```python
from build123d import *

# Parameters (mm, degrees)
BOX_W             = 5
BOX_H             = 6
BOX_DEPTH         = 8
CYLINDER001_R     = 1.675
CYLINDER001_DEPTH = 8


with BuildPart() as d:
    # Box → Box (new body)
    with BuildSketch(Plane(origin=(1, -3, 15), x_dir=(1, 0, 0), z_dir=(0, 0, 1))):
        with Locations((2.5, 3)):
            Rectangle(BOX_W, BOX_H)
    extrude(amount=BOX_DEPTH)


with BuildPart() as eje_d:
    # Cylinder001 → Cylinder001 (new body)
    with BuildSketch(Plane.XY.offset(15)):
        Circle(CYLINDER001_R)
    extrude(amount=CYLINDER001_DEPTH)

    # Cut: cut D
    add(d.part, mode=Mode.SUBTRACT)


with BuildPart() as eje_d_1:
    # Cut placement: moved
    add(eje_d.part.moved(Location((0, 0, -12))))


with BuildPart() as cut001:
    # Sketch → Revolution (revolve)
    with BuildSketch(Plane.XZ):
        Polygon((9.5, 11), (0, 11), (0, 0), (9.5, 0), (9.5, 0.5), (10, 0.5), (10, 10.5), (9.5, 10.5), align=None)
    revolve(axis=Axis((0, 0, 0), (0, 0, 1)))

    # Cut001: cut EJE + D
    add(eje_d_1.part, mode=Mode.SUBTRACT)


solid = cut001.part
```
Check sheet for the modelled part. Datum: model origin and axes. Units: mm. A direction names the side the tool comes from. Give positions to 0.01 mm unless a question says otherwise; leave off trailing zeros. Order: outer loops, then holes, each group sorted by start corner. A loop starts at its lowest first (then second) coordinate and runs counter-clockwise, first axis right, second up. Notation, with made-up numbers: (66.5, -5) -> (79.5, -5) arc R25 ccw to (79.5, 23) -> close; hole circle Ø5 at (-34, 1.5). An arc over 180 degrees is marked (long way). Return JSON: item names as keys, results as strings.
1. Set-up check for faces 5 (the flat face through (0, 0, 3)), 6 (the cylindrical face through (4.38, -8.43, 0.25)), 7 (the cylindrical face through (-2.17, -9.76, 5.57)): record each of +Z, -Z, +X, -X, +Y, -Y from which the full face is reachable in a straight line by a thin tool's end or side.
From the geometry:
{"face 5": "+Z", "face 6": "-Z", "face 7": "+Z, -Z"}
2. Mould release check, pull along Y, two halves, no side actions. Record for faces 1 (the flat face through (1, 0, 7)), 2 (the cylindrical face through (-1.674, 0.052, 6.944)), 3 (the flat face through (0, 0, 0)), 4 (the cylindrical face through (4.38, -8.43, 10.75)): +Y half, -Y half, draft (parallel to the pull), parting line (faces both ways), or undercut.
From the geometry:
{"face 1": "undercut", "face 2": "undercut", "face 3": "draft", "face 4": "parting line"}
3. Material ranges on probe 1 along Y at (x, z) = (0, 8) (3 decimals); probe 2 along X at (y, z) = (-2.25, 4); probe 3 along Y at (x, z) = (3, 3.5), recorded low to high. Write a range as [from, to].
From the geometry:
{"probe 1": "[-10, -1.675], [1.675, 10]", "probe 2": "[-9.74, 9.74]", "probe 3": "[-9.54, 9.54]"}
4. Cross-section at C-C, the plane z = 8.25. Record the cut outline in (x, y) (3 decimals).
From the geometry:
{"outline": "circle Ø20 at (0, 0); hole (1, -1.344) -> (1, 1.344) arc R1.675 ccw (long way) to start"}
5. Go/stop test with flat-tipped pins: P1, Ø5, axis at y = -3.5, z = 6.5, coming from the -X side; P2, Ø5, axis at x = 3, z = 3.5, coming from the -Y side; P3, Ø1, axis at x = -3.5, z = 2.5, coming from the +Y side. Record where each tip stops, or that it passes through.
From the geometry:
{"P1": "x = -9.95", "P2": "y = -9.99", "P3": "y = 9.54"}
6. Cross-section at D-D, the plane z = 2.25. Record the cut outline in (x, y).
From the geometry:
{"outline": "circle Ø20 at (0, 0)"}
7. Cross-section at B-B, the plane y = 0. Record the cut outline in (x, z) (3 decimals).
From the geometry:
{"outline": "(-10, 0.5) -> (-9.5, 0.5) -> (-9.5, 0) -> (9.5, 0) -> (9.5, 0.5) -> (10, 0.5) -> (10, 10.5) -> (9.5, 10.5) -> (9.5, 11) -> (1, 11) -> (1, 3) -> (-1.675, 3) -> (-1.675, 11) -> (-9.5, 11) -> (-9.5, 10.5) -> (-10, 10.5) -> close"}
8. Cross-section at A-A, the plane x = 0. Record the cut outline in (y, z) (3 decimals), plus the area to 3 significant figures.
From the geometry:
{"outline": "(-10, 0.5) -> (-9.5, 0.5) -> (-9.5, 0) -> (9.5, 0) -> (9.5, 0.5) -> (10, 0.5) -> (10, 10.5) -> (9.5, 10.5) -> (9.5, 11) -> (1.675, 11) -> (1.675, 3) -> (-1.675, 3) -> (-1.675, 11) -> (-9.5, 11) -> (-9.5, 10.5) -> (-10, 10.5) -> close", "area": "192 mm^2"}
